Can you work these out from the model? Positions are in its coordinate system, mm. Give positions to 0.01 mm unless a question says otherwise; leave off trailing zeros. Write each loop counter-clockwise with the first axis right and the second up, starting at its lowest first coordinate (ties: lowest second). Pieces come first, ordered by that corner, then holes.
from build123d import *

# Parameters (mm, degrees)
BOSS_EXTRUDE1_DEPTH = 3
CHAMFER6_SIZE       = 1.5
CHAMFER6_SIZE_2     = 3
CHAMFER7_SIZE       = 1.5
CHAMFER7_SIZE_2     = 3
CHAMFER8_SIZE       = 10
CHAMFER8_SIZE_2     = 1.5
CHAMFER9_SIZE       = 10
CHAMFER9_SIZE_2     = 1.5


with BuildPart() as part:
    # Sketch1 → Boss-Extrude1 (new body)
    with BuildSketch(Plane.XY):
        Polygon((76, 560.990034), (176, 380.990034), (176, 330.990034), (60.272319057, 300.990034), (0, 300.990034), (0, 560.990034), align=None)
    extrude(amount=BOSS_EXTRUDE1_DEPTH)

    # Sketch2 → Cut-Revolve1 (revolve, cut)
    with BuildSketch(Plane.XY.offset(1.5)):
        with BuildLine():
            Line((76, 500), (76, 585.578863385))
            Line((76, 585.578863385), (0, 585.578863385))
            Line((0, 585.578863385), (0, 0))
            add(Edge.make_bspline(
                [(0, 0), (0.013783816, 0.003488157), (0.04033603, 0.01319051), (0.089619378, 0.042063455), (0.174781236, 0.103253354), (0.279068591, 0.195655925), (0.394476748, 0.312893359), (0.511330855, 0.444471001), (0.661995475, 0.626416713), (0.874340043, 0.905417524), (1.210288344, 1.39310301), (1.747935993, 2.271497179), (2.58108843, 3.81588258), (3.907734136, 6.629844229), (5.990626535, 11.732179856), (8.974782838, 20.21551767), (12.492116493, 31.724489027), (16.281172086, 45.606799288), (21.020860811, 64.651371321), (26.206631662, 87.658368898), (31.746320492, 114.722363422), (37.537896498, 145.854010301), (42.871807206, 177.066921726), (47.80723428, 208.345145014), (52.381191067, 239.678124678), (56.615153522, 271.058803785), (60.519680025, 302.482154914), (63.648418258, 330.011833268), (66.11894295, 353.631593101), (68.030132581, 373.329466343), (69.466784443, 389.09643856), (70.806129018, 404.87199461), (71.886996993, 418.683052253), (72.742662769, 430.526418849), (73.404435972, 440.399441684), (73.901071328, 448.299980017), (74.304775576, 455.214817724), (74.62677953, 461.143160456), (74.877801518, 466.084350078), (75.067577987, 470.037846817), (75.336303636, 476.005510657), (75.563352259, 481.736537174), (75.748085722, 487.230769759), (75.884662604, 492.488061525), (75.940348523, 495.116996281), (75.978043797, 497.370577281), (75.993594118, 498.87307617), (76, 499.624354134), (76, 500)],
                knots=[0, 0, 0, 0, 0, 0.000111673, 0.000223346, 0.000446692, 0.000826683, 0.001206674, 0.00151955, 0.001832426, 0.00268779, 0.00396812, 0.006183448, 0.009942812, 0.016507085, 0.02846832, 0.049586633, 0.080772227, 0.111303184, 0.141834141, 0.204203935, 0.266574069, 0.32894426, 0.39131442, 0.453684463, 0.516054568, 0.578424701, 0.640794795, 0.703164955, 0.734350023, 0.765535092, 0.796720055, 0.827905019, 0.859090157, 0.874682727, 0.890275296, 0.905867787, 0.921460278, 0.929256523, 0.937052769, 0.944849014, 0.95264526, 0.97632263, 0.982241972, 0.988161315, 0.994080657, 0.997040329, 1, 1, 1, 1, 1], degree=4))
        make_face()
    revolve(axis=Axis((0, 0, 1.5), (0, 1, 0)), mode=Mode.SUBTRACT)

    # Chamfer6
    # the kernel refuses this chamfer: 3, 1.5 mm, written as the material it takes off along each edge
    with BuildSketch(Plane(origin=(72.226803743, 567.781787262, 3), x_dir=(0.060245471517658, 0.03346970639869887, -0.9976223042390342), z_dir=(0.4856429311786319, -0.8741572761215379, 0))) as chamfer6_piece_1:
        Polygon((CHAMFER6_SIZE * 0.997622304239, -CHAMFER6_SIZE * 0.0689183436017), (-CHAMFER6_SIZE_2 * 0.0689183436017, -CHAMFER6_SIZE_2 * 0.997622304239), (0, 0), align=None)
    extrude(amount=221.451576062, mode=Mode.SUBTRACT)

    # Chamfer7
    # the kernel refuses this chamfer: 3, 1.5 mm, written as the material it takes off along each edge
    with BuildSketch(Plane(origin=(72.226803743, 567.781787262, 0), x_dir=(0.060245471517658, 0.03346970639869887, 0.9976223042390342), z_dir=(0.4856429311786319, -0.8741572761215379, 0))) as chamfer7_piece_1:
        Polygon((CHAMFER7_SIZE * 0.997622304239, CHAMFER7_SIZE * 0.0689183436017), (-CHAMFER7_SIZE_2 * 0.0689183436017, CHAMFER7_SIZE_2 * 0.997622304239), (0, 0), align=None)
    extrude(amount=221.451576062, mode=Mode.SUBTRACT)

    # Chamfer8
    # the kernel refuses this chamfer: 10, 1.5 mm, written as the material it takes off along each edge
    with BuildSketch(Plane(origin=(201.157802967, 337.511672409, 3), x_dir=(-0.250930852134312, 0.9679881864854557, 0.005707737883485932), z_dir=(-0.9680039545618228, -0.2509349396809314, 0))) as chamfer8_piece_1:
        Polygon((CHAMFER8_SIZE * 0.999983710731, CHAMFER8_SIZE * 0.00570773788349), (-CHAMFER8_SIZE_2 * 0.00570773788349, CHAMFER8_SIZE_2 * 0.999983710731), (0, 0), align=None)
    extrude(amount=171.531620397, mode=Mode.SUBTRACT)

    # Chamfer9
    # the kernel refuses this chamfer: 10, 1.5 mm, written as the material it takes off along each edge
    with BuildSketch(Plane(origin=(201.157802967, 337.511672409, 0), x_dir=(-0.250930852134312, 0.9679881864854557, -0.005707737883485934), z_dir=(-0.9680039545618228, -0.2509349396809314, 0))) as chamfer9_piece_1:
        Polygon((CHAMFER9_SIZE * 0.999983710731, -CHAMFER9_SIZE * 0.00570773788349), (-CHAMFER9_SIZE_2 * 0.00570773788349, -CHAMFER9_SIZE_2 * 0.999983710731), (0, 0), align=None)
    extrude(amount=171.531620397, mode=Mode.SUBTRACT)


solid = part.part
(1) Will this pin go through, and if not, where does the flat tip stop? P1, Ø1.5, axis at x = 112, z = 1, coming from the +Y side.
Returned:
P1: stops at y = 497.2
(2) Imagine slicing it at C-C, the plane x = 97. Write out the boundary of the cut face in (y, z).
Returned:
outline: (310.51, 1.5) - (320.84, 0) - (517.01, 0) - (523.19, 1.5) - (517.01, 3) - (320.84, 3) - close
(3) Imagine slicing it at B-B, the plane x = 153. Write out the boundary of the cut face in (y, z), plus the area to 3 significant figures.
Returned:
outline: (325.03, 1.5) - (335.36, 0) - (416.21, 0) - (422.39, 1.5) - (416.21, 3) - (335.36, 3) - close
area: 267 mm2
(4) Imagine slicing it at A-A, the plane y = 540. Write out the boundary of the cut face in (x, z).
Returned:
outline: (75.99, 0) - (84.23, 0) - (87.66, 1.5) - (84.23, 3) - (75.99, 3) arc R76 cw to start
(5) If I drill on L1, parallel to X at y = 471, z = 1.4; L2, parallel to X at y = 450.5, z = 1.25, over which ranges is the centre line in solid material (lowest first)?
Returned:
L1: x = 75.11 to 125.77
L2: x = 74.03 to 136.81
